Input: part model. Units: mm. Frame: model coordinates. Coordinates: 2 decimals unless noted, no trailing zeros. Write each loop counter-clockwise with the first axis right and the second up, starting at its lowest first coordinate (ties: lowest second). Pieces come first, ordered by that corner, then holes. Notation, with made-up numbers: (5, 59) -> (37, 59) arc R13 ccw to (37, 73) -> close; hole circle Ø1 at (30, 36). An arc over 180 degrees is marked (long way). Use one line per item in the form item = value. Start each with the question number.
(1) Cut plane B-B on x = -41. Return the cut outline in (y, z), plus the area to 4 significant figures.
(2) First-contact query: pin 1 (0.8 mm diameter, centred on x = 40, z = 1.5, fed in from -Y). Flat tip, straight axial feed; report the tip coordinate or a pass-through.
(3) Cut plane A-A on z = 0.8. Return the cut outline in (x, y), plus the area to 3 significant figures.
(4) Ray query, line 1 along X through (y, z) = (23, 0.45); line 2 along Y through (x, z) = (35.5, 1.9). Return the intervals inside material, ascending.
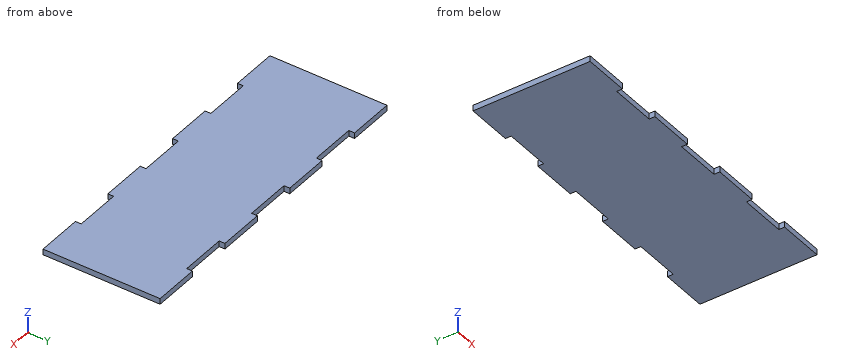
```python
from build123d import *

# Parameters (mm, degrees)
SKETCH1_W           = 139.7
SKETCH1_H           = 50.8
BOSS_EXTRUDE1_DEPTH = 2.5
SKETCH3_W           = 19.957142857
SKETCH3_H           = 2.5
SKETCH3_W_2         = 19.957142858
CUT_EXTRUDE2_DEPTH  = 2.54


with BuildPart() as part:
    # Sketch1 → Boss-Extrude1 (new body)
    with BuildSketch(Plane.XY):
        Rectangle(SKETCH1_W, SKETCH1_H)
    extrude(amount=BOSS_EXTRUDE1_DEPTH)

    # Sketch3 → Cut-Extrude2 (cut)
    with BuildSketch(Plane(origin=(0, 0, 0), x_dir=(-1, 0, 0), z_dir=(0, 0, -1))):
        with Locations((-39.914285715, 24.15)):
            Rectangle(SKETCH3_W, SKETCH3_H)
        with Locations((0, 24.15)):
            Rectangle(SKETCH3_W_2, SKETCH3_H)
        with Locations((39.914285715, 24.15)):
            Rectangle(SKETCH3_W, SKETCH3_H)
        with Locations((-39.914285715, -24.15)):
            Rectangle(SKETCH3_W, SKETCH3_H)
        with Locations((0, -24.15)):
            Rectangle(SKETCH3_W_2, SKETCH3_H)
        with Locations((39.914285715, -24.15)):
            Rectangle(SKETCH3_W, SKETCH3_H)
    extrude(amount=-CUT_EXTRUDE2_DEPTH, mode=Mode.SUBTRACT)


solid = part.part
```
Values:
q1.outline = (-22.9, 0) -> (22.9, 0) -> (22.9, 2.5) -> (-22.9, 2.5) -> close
q1.area = 114.5 mm2
q2.pin_1 = -22.9
q3.outline = (-69.85, -25.4) -> (-49.89, -25.4) -> (-49.89, -22.9) -> (-29.94, -22.9) -> (-29.94, -25.4) -> (-9.98, -25.4) -> (-9.98, -22.9) -> (9.98, -22.9) -> (9.98, -25.4) -> (29.94, -25.4) -> (29.94, -22.9) -> (49.89, -22.9) -> (49.89, -25.4) -> (69.85, -25.4) -> (69.85, 25.4) -> (49.89, 25.4) -> (49.89, 22.9) -> (29.94, 22.9) -> (29.94, 25.4) -> (9.98, 25.4) -> (9.98, 22.9) -> (-9.98, 22.9) -> (-9.98, 25.4) -> (-29.94, 25.4) -> (-29.94, 22.9) -> (-49.89, 22.9) -> (-49.89, 25.4) -> (-69.85, 25.4) -> close
q3.area = 6,800 mm2
q4.line_1 = -69.85 to -49.89, -29.94 to -9.98, 9.98 to 29.94, 49.89 to 69.85
q4.line_2 = -22.9 to 22.9
